Can you work these out from the model? Positions are in its coordinate system, mm. A direction names the side the tool comes from. Coordinates: 2 decimals unless noted, no trailing zeros. Order: outer loops, then holes, each group sorted by start corner. A loop starts at its lowest first (then second) coordinate and runs counter-clockwise, first axis right, second up. Notation, with made-up numbers: (-30, 8) -> (-20, 8) arc R32 ccw to (-20, 47) -> close; hole circle Ø1 at (55, -2). An arc over 180 degrees is marked (long way). Return JSON: item names as keys, results as strings. Group by question number.
1) If we section it at C-C, the plane x = 2.25: Please give me the cut outline in (y, z) (3 decimals).
2) If we section it at B-B, the plane z = 1.25: Please give me the cut outline in (x, y), then the cut area to 3 significant figures.
3) If I drill on probe 1 along X at (y, z) = (-2.5, -1); probe 2 along Y at (x, z) = (0, -1.75); probe 3 along Y at (x, z) = (5, -0.5), over which ranges is the centre line in solid material (lowest first)? Write a range as from..to.
4) For faces 1 (the cylindrical face through (6.799, 2.508, -0.79)), 2 (the flat face through (9.017, 0, 0)), which set-ups out of +Z, -Z, +X, -X, +Y, -Y let a thin tool reach every point of the face, with its end or its side?
5) If we section it at A-A, the plane y = 0.5: Please give me the cut outline in (x, z), then the cut area to 3 significant figures.
6) Thinking about a two-plate mould opening in X: for faces 3 (the flat face through (6.477, 0, -3)), 4 (the flat face through (-6.477, 0, -3)), 5 (the flat face through (-9.017, 0, 0)), 6 (the cylindrical face through (8.08, 0.95, -3.03)), which applies, +X half, -X half, draft (parallel to the pull), parting line (faces both ways), or undercut?
from build123d import *

# Parameters (mm, degrees)
SKETCH1_R      = 3.175
EXTRUDE1_DEPTH = 9.017
SKETCH2_W      = 0.635
SKETCH2_H      = 0.5461


with BuildPart() as part:
    # Sketch1 → Extrude1 (new body, symmetric)
    with BuildSketch(Plane(origin=(0, 0, 0), x_dir=(0, 0, -1), z_dir=(1, 0, 0))):
        Circle(SKETCH1_R)
    extrude(amount=EXTRUDE1_DEPTH, both=True)

    # Sketch2 → Cut-Revolve1 (revolve, cut)
    with BuildSketch(Plane.XY):
        with Locations((-6.7945, 2.90195)):
            Rectangle(SKETCH2_W, SKETCH2_H)
        with Locations((6.7945, 2.90195)):
            Rectangle(SKETCH2_W, SKETCH2_H)
    revolve(axis=Axis((0, 0, 0), (-1, 0, 0)), mode=Mode.SUBTRACT)


solid = part.part
Result sheet:
{
 "1": {"outline": "circle Ø6.35 at (0, 0)"},
 "2": {"outline": "(-9.02, -2.92) -> (-7.11, -2.92) -> (-7.11, -2.31) -> (-6.48, -2.31) -> (-6.48, -2.92) -> (6.48, -2.92) -> (6.48, -2.31) -> (7.11, -2.31) -> (7.11, -2.92) -> (9.02, -2.92) -> (9.02, 2.92) -> (7.11, 2.92) -> (7.11, 2.31) -> (6.48, 2.31) -> (6.48, 2.92) -> (-6.48, 2.92) -> (-6.48, 2.31) -> (-7.11, 2.31) -> (-7.11, 2.92) -> (-9.02, 2.92) -> close", "area": "104 mm2"},
 "3": {"probe 1": "x = -9.02..-7.11, -6.48..6.48, 7.11..9.02", "probe 2": "y = -2.65..2.65", "probe 3": "y = -3.14..3.14"},
 "4": {"face 1": "none", "face 2": "+Z, -Z, +X, +Y, -Y"},
 "5": {"outline": "(-9.02, -3.14) -> (-7.11, -3.14) -> (-7.11, -2.58) -> (-6.48, -2.58) -> (-6.48, -3.14) -> (6.48, -3.14) -> (6.48, -2.58) -> (7.11, -2.58) -> (7.11, -3.14) -> (9.02, -3.14) -> (9.02, 3.14) -> (7.11, 3.14) -> (7.11, 2.58) -> (6.48, 2.58) -> (6.48, 3.14) -> (-6.48, 3.14) -> (-6.48, 2.58) -> (-7.11, 2.58) -> (-7.11, 3.14) -> (-9.02, 3.14) -> close", "area": "112 mm2"},
 "6": {"face 3": "undercut", "face 4": "undercut", "face 5": "-X half", "face 6": "draft"}
}
